Autodesk Inventor part; units mm, degrees
ref_plane "Work Plane1" through (-9, 33.5885, 16.5511) normal (1, 0, 0) x (0, 0, -1)
ref_plane "YZ Plane" through (0, 0, 0) normal (1, 0, 0) x (0, 1, 0)
ref_plane "XZ Plane" through (0, 0, 0) normal (0, 1, 0) x (-1, 0, 0)
sketch "Sketch1" plane through (0, 0, 0) normal (0, 1, 0) x (-1, 0, 0)
  line L0 (0, 0) -> (18, 0)
  line L1 (18, 0) -> (18, 18)
  line L2 (18, 18) -> (0, 18)
  line L3 (0, 18) -> (0, 0)
  dimension "d0" = 18
  dimension "d1" = 18
extrude "Extrusion1" add sketch "Sketch1" along normal blind 8 draft -15
fillet "Fillet1" radius 1.5 8 edges at (-1.0718, 4, 16.9282) (-9, 8, 15.8564) (-2.1436, 8, 9) (-9, 8, 2.1436) (-1.0718, 4, 1.0718) (-16.9282, 4, 1.0718) (-16.9282, 4, 16.9282) (-15.8564, 8, 9)
ref_plane "Work Plane1" through (-9, 33.5885, 16.5511) normal (1, 0, 0) x (0, 0, -1)
sketch "Sketch2" plane through (-9, 33.5885, 16.5511) normal (1, 0, 0) x (0, 0, -1)
  line L0 (13.2565, -25.5885) -> (1.8457, -25.5885)
  arc A0 (14.7054, -26.7002) -> (13.2565, -25.5885) centre (13.2565, -27.0885) ccw
  arc A1 (1.8457, -25.5885) -> (13.2565, -25.5885) centre (7.5511, -15.0316) ccw
  point P0 (16.5511, -33.5885)
  point P1 (13.2565, -25.5885)
  dimension "d5" = 12
extrude "Extrusion2" cut sketch "Sketch2" along normal through all both and the other way through all
sketch "Sketch3" plane through (0, 0, 0) normal (0, -1, 0) x (1, 0, 0)
  line L0 (-16.5511, 18) -> (-1.4489, 18) construction
  line L1 (-9, 18) -> (-9, 0) construction
  line L2 (-1.4489, 0) -> (-16.5511, 0) construction
  line L3 (-18, 1.4489) -> (-18, 16.5511) construction
  line L4 (-18, 9) -> (0, 9) construction
  line L5 (-1, 1) -> (-17, 1)
  line L6 (-17, 1) -> (-17, 17)
  line L7 (-17, 17) -> (-1, 17)
  line L8 (-1, 17) -> (-1, 1)
  line L9 (-1, 1) -> (-17, 17) construction
  line L10 (-17, 1) -> (-1, 17) construction
  point P0 (0, 0)
  point P1 (-9, 9)
  point P2 (-9, 9)
  dimension "d8" = 16
  dimension "d9" = 16
extrude "Extrusion3" cut sketch "Sketch3" against normal blind 4.5 draft -15
sketch "Sketch4" plane through (0, 4.5, 0) normal (0, -1, 0) x (1, 0, 0)
  line L0 (-15.7942, 15.7942) -> (-15.7942, 2.2058) construction
  line L1 (-15.7942, 9) -> (-2.2058, 9) construction
  line L2 (-2.2058, 2.2058) -> (-2.2058, 15.7942) construction
  line L3 (-2.2058, 15.7942) -> (-15.7942, 15.7942) construction
  line L4 (-9, 15.7942) -> (-9, 2.2058) construction
  line L5 (-15.7942, 2.2058) -> (-2.2058, 2.2058) construction
  circle A0 centre (-9, 9) radius 2.775
  point P0 (0, 0)
  dimension "d12" = 5.55
extrude "Extrusion4" add sketch "Sketch4" along normal blind 4
sketch "Sketch5" plane through (-9, 0.5, 9) normal (0, -1, 0) x (1, 0, 0)
  line L0 (1.5875, 2.075) -> (-1.5875, 2.075)
  line L1 (-1.5875, -2.075) -> (1.5875, -2.075)
  line L2 (-1.5875, 2.075) -> (1.5875, -2.075) construction
  line L3 (-2.075, 1.5875) -> (-2.075, -1.5875)
  line L4 (2.075, -1.5875) -> (2.075, 1.5875)
  line L5 (2.075, 1.5875) -> (-2.075, -1.5875) construction
  line L6 (-2.075, 1.5875) -> (2.075, -1.5875) construction
  line L7 (-6.7942, 6.7942) -> (-6.7942, -6.7942) construction
  line L8 (-6.7942, 0) -> (6.7942, 0) construction
  line L9 (6.7942, -6.7942) -> (6.7942, 6.7942) construction
  line L10 (-6.7942, -6.7942) -> (6.7942, -6.7942) construction
  line L11 (0, -6.7942) -> (0, 6.7942) construction
  line L12 (-1.5875, 2.075) -> (-1.5875, 1.8875)
  line L13 (-1.5875, -1.8875) -> (-1.5875, -2.075)
  line L14 (-2.075, -1.5875) -> (-1.8875, -1.5875)
  line L15 (-1.8875, 1.5875) -> (-2.075, 1.5875)
  line L16 (0, 0) -> (-1.5875, -2.075) construction
  line L17 (2.075, 1.5875) -> (1.8875, 1.5875)
  line L18 (1.8875, -1.5875) -> (2.075, -1.5875)
  line L19 (1.5875, -2.075) -> (1.5875, -1.8875)
  line L20 (1.5875, 1.8875) -> (1.5875, 2.075)
  line L21 (-1.5875, 1.8875) -> (-1.5875, -1.8875)
  line L22 (1.8875, 1.5875) -> (1.5875, 1.5875)
  line L23 (-1.5875, 1.5875) -> (-1.8875, 1.5875)
  line L24 (1.5875, -1.8875) -> (1.5875, -1.5875)
  line L25 (1.5875, 1.2145) -> (1.5875, 1.8875)
  line L26 (1.8875, -1.5875) -> (1.5875, -1.5875)
  line L27 (-1.5875, -1.5875) -> (-1.8875, -1.5875)
  point P0 (9, -9)
  dimension "d15" = 3.175
  dimension "d16" = 4.15
  dimension "d17" = 4.15
  dimension "d18" = 3.175
extrude "Extrusion5" cut sketch "Sketch5" against normal blind 4
properties part number "Keycap"
Verification items for the finished model (mm, model axes). A direction names the side the tool comes from. Give positions to 0.01 mm unless a question says otherwise; leave off trailing zeros. Loops run counter-clockwise (first coordinate to the right, second up) from the corner with the lowest first, then second, coordinate; pieces in that order, holes last. Notation, with made-up numbers: M 85.25,53 L 129.25,53 A28 ccw 129.25,76 Z; hole C -16,-20.75 d1. An arc over 180 degrees is marked long. Return JSON: item names as keys, results as strings.
1) Section check B-B, the plane z = 9. Enter the section's corners in (x, y) (3 decimals).
Findings:
{"outline": "M -18,0 L -17,0 L -15.794,4.5 L -11.775,4.5 L -11.775,0.5 L -11.075,0.5 L -11.075,4.5 L -6.925,4.5 L -6.925,0.5 L -6.225,0.5 L -6.225,4.5 L -2.206,4.5 L -1,0 L 0,0 L -1.757,6.557 L -16.243,6.557 Z"}
2) Material ranges on L1, parallel to Z at x = -9.5, y = 1.25 (3 decimals); L2, parallel to Z at x = -6.5, y = 0.75; L3, parallel to X at y = 0.75, z = 7.5 (3 decimals), recorded low to high. Write a range as [from, to].
Findings:
{"L1": "z = [0.335, 1.335], [6.27, 6.925], [11.075, 11.73], [16.665, 17.665]", "L2": "z = [0.2, 1.2], [7.8, 10.2], [16.8, 17.8]", "L3": "x = [-17.799, -16.799], [-11.335, -11.075], [-6.925, -6.665], [-1.201, -0.201]"}
3) Section check A-A, the plane x = -9. Enter the section's corners in (y, z) (3 decimals), and give its area (3 significant figures).
Findings:
{"outline": "M 0,0 L 6.888,1.846 A1.5 ccw 8,3.295 A12 cw 8,14.705 A1.5 ccw 6.888,16.154 L 0,18 L 0,17 L 4.5,15.794 L 4.5,11.775 L 0.5,11.775 L 0.5,11.075 L 4.5,11.075 L 4.5,6.925 L 0.5,6.925 L 0.5,6.225 L 4.5,6.225 L 4.5,2.206 L 0,1 Z", "area": "54.3 mm2"}
4) Section check D-D, the plane x = -3.75. Enter the section's corners in (y, z).
Findings:
{"outline": "M 0,0 L 6.89,1.85 A1.5 ccw 8,3.29 A12 cw 8,14.71 A1.5 ccw 6.89,16.15 L 0,18 L 0,17 L 4.5,15.79 L 4.5,2.21 L 0,1 Z"}
5) Gauge pin test, flat ends, axial feed: P1, Ø1, axis at y = 2, z = 8, coming from the -X side; P2, Ø10, axis at x = -13.5, z = 9, coming from the +Y side; P3, Ø1, axis at x = -9.5, y = 2.5, coming from the -Z side. Record the tip position at first contact, or that the pin passes through.
Findings:
{"P1": "stops at x = -17.6", "P2": "stops at y = 7.65", "P3": "stops at z = 0.54"}
6) Mould release check, pull along X, two halves, no side actions. Record for faces 1 (the flat face through (-9.11, 3.4, 17.09)), 2 (the cylindrical face through (-16.637, 3.565, 16.615)), 3 (the flat face through (-1.594, 2.218, 9.112)): released by +X, released by -X, zero draft, split by the parting line, or undercut.
Findings:
{"face 1": "zero draft", "face 2": "released by -X", "face 3": "undercut"}
7) Section check C-C, the plane y = 3.25. Count the separate pieces of the cut face and the enclosed holes in it, and give its area (3 significant figures).
Findings:
{"separate pieces": "2", "enclosed holes": "2", "area": "67.2 mm2"}
8) Tool access check on faces 4 (the cylindrical face through (-1.385, 3.565, 16.637)), 5 (the flat face through (-9.22, 0.5, 6.75)). Record the directions out of +Z, -Z, +X, -X, +Y, -Y that give a thin tool (end or side, any length) a straight path to the whole face; none if there is none.
Findings:
{"face 4": "+Z, +X, +Y", "face 5": "-Y"}
